from build123d import *

# Parameters (mm, degrees)
BOSS_EXTRUDE1_DEPTH = 50
SKETCH3_W           = 14.282150027
SKETCH3_H           = 50
BOSS_EXTRUDE2_DEPTH = 100
CUT_EXTRUDE1_START  = -200
SKETCH4_R           = 55
CUT_EXTRUDE1_DEPTH  = 200


with BuildPart() as part:
    # Sketch1 → Boss-Extrude1 (new body)
    with BuildSketch(Plane(origin=(0, 0, 0), x_dir=(1, 0, 0), z_dir=(0, 1, 0))):
        with BuildLine():
            ThreePointArc((-70, 0), (0, -70), (70, 0))
            Line((70, 0), (55, 0))
            ThreePointArc((55, 0), (0, -55), (-55, 0))
            Line((-55, 0), (-70, 0))
        make_face()
    extrude(amount=BOSS_EXTRUDE1_DEPTH)

    # Sketch3 → Boss-Extrude2 (add, symmetric)
    with BuildSketch(Plane(origin=(0, 0, 0), x_dir=(0, 0, -1), z_dir=(1, 0, 0))):
        with Locations((-7.141075014, 25)):
            Rectangle(SKETCH3_W, SKETCH3_H)
    extrude(amount=BOSS_EXTRUDE2_DEPTH, both=True)

    # Sketch4 → Cut-Extrude1 (cut)
    with BuildSketch(Plane(origin=(0, 50, 0), x_dir=(1, 0, 0), z_dir=(0, 1, 0)).offset(CUT_EXTRUDE1_START)):
        Circle(SKETCH4_R)
    extrude(amount=CUT_EXTRUDE1_DEPTH, mode=Mode.SUBTRACT)


solid = part.part
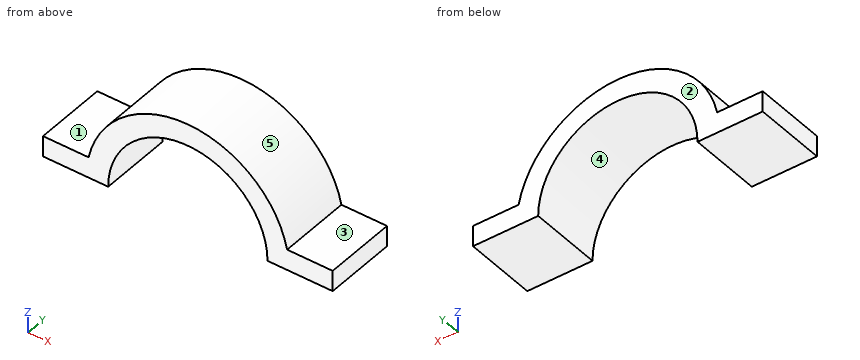
Design review of the part built by this model. Coordinates are the model's own, in mm. Face numbers are marked on the shaded views. A direction names the side the tool comes from. Round coordinates to 2 decimals unless told otherwise and drop trailing zeros. Write each loop counter-clockwise with the first axis right and the second up, starting at its lowest first coordinate (ties: lowest second). Pieces come first, ordered by that corner, then holes.
Item 1: Wall thickness on L1, parallel to X at y = 45.5, z = 32.5; L2, parallel to X at y = 46.5, z = 14; L3, parallel to Z at x = 91, y = 21: over which ranges is each line inside the solid? List them lowest first.
Item 2: Consider section C-C on z = 64. Give the boundary of the cut face in (x, y), and give its area (3 significant figures).
Item 3: Consider section B-B on x = 0. Give the boundary of the cut face in (y, z), and give its area (3 significant figures).
Item 4: For pin 1 Ø1.5 at (x, y) = (6.5, 34.5) entering from +Z; pin 2 Ø2 at (y, z) = (8.5, 21.5) entering from -X; pin 3 Ø2 at (x, y) = (-61.5, 34) entering from +Z, all flat-tipped, find the tip position at first contact; note any pin that passes through.
Item 5: Draft analysis for pull direction X (two halves, no side actions). For the marked faces 3, 4 and 5, state which applies: released by +X, released by -X, zero draft, split by the parting line, or undercut.
Item 6: For the marked faces 1 and 2, list the 3-axis set-ups (+Z, -Z, +X, -X, +Y, -Y) from which the entire face can be reached by the end or side of a thin tool; tool diameter is ignored.
Item 7: Consider section A-A on y = 12.5. Give the boundary of the cut face in (x, z), and give its area (3 significant figures).
Check values:
1. L1: x = -62 to -44.37, 44.37 to 62
1. L2: x = -100 to -53.19, 53.19 to 100
1. L3: z = 0 to 14.28
2. outline: (-28.35, 0) - (28.35, 0) - (28.35, 50) - (-28.35, 50) - close
2. area: 2,840 mm2
3. outline: (0, 55) - (50, 55) - (50, 70) - (0, 70) - close
3. area: 750 mm2
4. pin 1: stops at z = 69.76
4. pin 2: stops at x = -66.93
4. pin 3: stops at z = 35.21
5. face 3: zero draft
5. face 4: undercut
5. face 5: split by the parting line
6. face 1: +Z, -X, +Y, -Y
6. face 2: +Z, -Z, +X, -X, +Y
7. outline: (-100, 0) - (-55, 0) arc R55 cw to (55, 0) - (100, 0) - (100, 14.28) - (68.53, 14.28) arc R70 ccw to (-68.53, 14.28) - (-100, 14.28) - close
7. area: 3,820 mm2
